CAD build for the part. Positions are in the model's coordinates, mm. Face numbers are marked on the shaded views. Coordinates: 2 decimals unless noted, no trailing zeros. Write each loop counter-clockwise with the first axis right and the second up, starting at its lowest first coordinate (ties: lowest second). Pieces come first, ordered by that corner, then holes. Notation, with made-up numbers: (26.5, 28.25) -> (63.5, 28.25) arc R23 cw to (63.5, 65.25) -> close; hole circle Ø6 at (58, 74.25). An arc over 180 degrees is marked (long way). Answer as CSV lines item,"result". Start each with the question number.
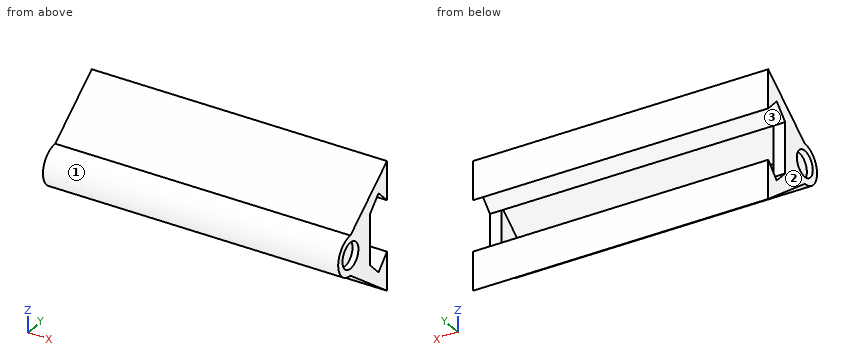
```python
from build123d import *

# Parameters (mm, degrees)
BOSS_EXTRUDE1_DEPTH = 15.875
SHELL1_START        = -14.605
SHELL1_DEPTH        = 29.21
SKETCH3_R           = 1.383918908
CUT_EXTRUDE2_DEPTH  = 0.635


# Read off the part's stored shape, not the designer's step: Shell1
with BuildPart() as part:
    # Sketch1 → Boss-Extrude1 (new, symmetric)
    with BuildSketch(Plane(origin=(0, 0, 0), x_dir=(0, 0, -1), z_dir=(1, 0, 0))):
        with BuildLine():
            Line((6.857311765, -3.076782348), (2.123637644, -9.426782348))
            ThreePointArc((2.123637644, -9.426782348), (0, -11.550419992), (-2.123637644, -9.426782348))
            Line((-2.123637644, -9.426782348), (-6.857311765, -3.076782348))
            Line((-6.857311765, -3.076782348), (-2.717266513, -3.076782348))
            Line((-2.717266513, -3.076782348), (-4.18616331, -4.545679146))
            Line((-4.18616331, -4.545679146), (-2.717266513, -6.014575943))
            Line((-2.717266513, -6.014575943), (2.717266513, -6.014575943))
            Line((2.717266513, -6.014575943), (4.18616331, -4.545679146))
            Line((4.18616331, -4.545679146), (2.717266513, -3.076782348))
            Line((2.717266513, -3.076782348), (6.857311765, -3.076782348))
        make_face()
    extrude(amount=BOSS_EXTRUDE1_DEPTH, both=True)

    # Shell1 outline → Shell1 (cut)
    with BuildSketch(Plane.YZ.offset(SHELL1_START)):
        with BuildLine():
            Line((-6.014575943, -3.083255099), (-6.014575943, 3.083255099))
            Line((-6.014575943, 3.083255099), (-9.095341146, 0.786666357))
            ThreePointArc((-9.095341146, 0.786666357), (-10.280419992, 0), (-9.095341146, -0.786666357))
            Line((-9.095341146, -0.786666357), (-6.014575943, -3.083255099))
        make_face()
    extrude(amount=SHELL1_DEPTH, mode=Mode.SUBTRACT)

    # Sketch3 → Cut-Extrude2 (cut)
    with BuildSketch(Plane.ZY.offset(15.875)):
        with Locations((0, -9.426782348)):
            Circle(SKETCH3_R)
    cut_extrude2 = extrude(amount=-CUT_EXTRUDE2_DEPTH, mode=Mode.SUBTRACT)

    # Mirror1: Cut-Extrude2 across plane
    add(cut_extrude2.mirror(Plane(origin=(0, 0, 0), x_dir=(0, 0, 1), z_dir=(1, 0, 0))), mode=Mode.SUBTRACT)


solid = part.part
```
1. Wall check: line 1 (Y direction, x = 15.45, z = 0); line 2 (X direction, y = -8.25, z = 1) (3 decimals); line 3 (X direction, y = -9.5, z = 0.5) (3 decimals). Give the ranges that are in metal, low to high.
2. Cut at B-B (z = 3.75). Give the cut face in (x, y) (3 decimals).
3. Cut at C-C (y = -3.5). Give the cut face in (x, z) (3 decimals), then the cut area to 3 significant figures.
4. Flat gauge pins, fed straight in: P1, Ø2.5, axis at y = -9.43, z = 0, coming from the -X side; P2, Ø5, axis at x = 3.5, y = -6.5, coming from the +Z side; P3, Ø4, axis at x = 11.5, y = -8, coming from the +Z side. Where does each tip first touch, or does it go through?
5. Cut at A-A (x = 2). Give the cut face in (y, z), then the cut area to 3 significant figures.
6. Cut at D-D (z = 0). Give the cut face in (x, y) (3 decimals).
7. Mould opens along Z. For the marked faces 1, 2 and 3 say: pulls with the +Z half, pulls with the -Z half, needs draft (parallel to the pull), parting line crosses it, or undercut.
Geometry check:
1,line 1,"-11.55 to -10.81, -8.04 to -6.01"
1,line 2,"-15.875 to -14.605, 14.605 to 15.875"
1,line 3,"-15.24 to -14.605, 14.605 to 15.24"
2,outline,"(-15.875, -7.245) -> (15.875, -7.245) -> (15.875, -4.982) -> (-15.875, -4.982) -> close; (-15.875, -4.11) -> (15.875, -4.11) -> (15.875, -3.077) -> (-15.875, -3.077) -> close"
3,outline,"(-15.875, -6.542) -> (15.875, -6.542) -> (15.875, -3.14) -> (-15.875, -3.14) -> close; (-15.875, 3.14) -> (15.875, 3.14) -> (15.875, 6.542) -> (-15.875, 6.542) -> close"
3,area,"216 mm²"
4,P1,"x = -15.24"
4,P2,"z = 6.17"
4,P3,"z = 4.68"
5,outline,"(-9.43, -2.12) -> (-3.08, -6.86) -> (-3.08, -2.72) -> (-4.55, -4.19) -> (-6.01, -2.72) -> (-6.01, -3.08) -> (-9.1, -0.79) arc R0.85 cw (long way) to (-9.1, 0.79) -> (-6.01, 3.08) -> (-6.01, 2.72) -> (-4.55, 4.19) -> (-3.08, 2.72) -> (-3.08, 6.86) -> (-9.43, 2.12) arc R2.12 ccw to start"
5,area,"30.2 mm²"
6,outline,"(-15.875, -11.55) -> (15.875, -11.55) -> (15.875, -10.811) -> (15.24, -10.811) -> (15.24, -8.043) -> (15.875, -8.043) -> (15.875, -6.015) -> (14.605, -6.015) -> (14.605, -10.28) -> (-14.605, -10.28) -> (-14.605, -6.015) -> (-15.875, -6.015) -> (-15.875, -8.043) -> (-15.24, -8.043) -> (-15.24, -10.811) -> (-15.875, -10.811) -> close"
7,face 1,"parting line crosses it"
7,face 2,"needs draft"
7,face 3,"undercut"
